from build123d import *

# Parameters (mm, degrees)
SKETCH_1_W          = 10
SKETCH_1_H          = 3
EXTRUDE_1_DEPTH     = 10
SKETCH_2_R          = 4.3
CUT_EXTRUDE_1_DEPTH = 11
SKETCH_3_R          = 1.75
CUT_EXTRUDE_2_DEPTH = 4
FILLET_1_R          = 3
FILLET_2_R          = 1


with BuildPart() as part:
    # ｽｹｯﾁ1 → ﾎﾞｽ - 押し出し1 (new body)
    with BuildSketch(Plane.XY):
        Polygon((7, 10), (1, 10), (1, -5), (7, -5), (7, 7), align=None)
        with Locations((12, 8.5)):
            Rectangle(SKETCH_1_W, SKETCH_1_H)
        Polygon((1, -5), (1, 10), (-5, 10), (-5, 7), (-5, -5), align=None)
        with Locations((-10, 8.5)):
            Rectangle(SKETCH_1_W, SKETCH_1_H)
    extrude(amount=EXTRUDE_1_DEPTH)

    # ｽｹｯﾁ2 → ｶｯﾄ - 押し出し1 (cut, through all)
    with BuildSketch(Plane(origin=(0, 0, 0), x_dir=(-1, 0, 0), z_dir=(0, 0, -1))):
        with Locations((-1, 1)):
            Circle(SKETCH_2_R)
    extrude(amount=-CUT_EXTRUDE_1_DEPTH, mode=Mode.SUBTRACT)

    # ｽｹｯﾁ3 → ｶｯﾄ - 押し出し2 (cut, through all)
    with BuildSketch(Plane.XZ.offset(-7)):
        with Locations((-11.5, 5)):
            Circle(SKETCH_3_R)
        with Locations((13.5, 5)):
            Circle(SKETCH_3_R)
    extrude(amount=-CUT_EXTRUDE_2_DEPTH, mode=Mode.SUBTRACT)

    # ﾌｨﾚｯﾄ1
    fillet_1_edges = [part.edges().sort_by_distance(p)[0] for p in [
        (7, -5, 5),
        (-5, -5, 5),
        (-5, 7, 5),
        (7, 7, 5),
    ]]
    fillet(fillet_1_edges, radius=FILLET_1_R)

    # ﾌｨﾚｯﾄ2
    fillet_2_edges = [part.edges().sort_by_distance(p)[0] for p in [
        (-15, 8.5, 0),
        (17, 8.5, 0),
        (17, 8.5, 10),
        (-15, 7, 5),
        (17, 7, 5),
        (-15, 8.5, 10),
        (-5, 1, 0),
        (-5, 1, 10),
        (-11.5, 7, 0),
        (-11.5, 7, 10),
        (13.5, 7, 0),
        (13.5, 7, 10),
        (7, 1, 0),
        (7, 1, 10),
        (1, -5, 0),
        (1, -5, 10),
        (6.121320344, -4.121320344, 0),
        (-4.121320344, -4.121320344, 0),
        (6.121320344, -4.121320344, 10),
        (-4.121320344, -4.121320344, 10),
        (-5.878679656, 6.121320344, 0),
        (-5.878679656, 6.121320344, 10),
        (7.878679656, 6.121320344, 0),
        (7.878679656, 6.121320344, 10),
    ]]
    fillet(fillet_2_edges, radius=FILLET_2_R)


solid = part.part
Work out the finished part from the listing and answer in its coordinate system (mm). A direction names the side the tool comes from. Give positions to 0.01 mm unless a question says otherwise; leave off trailing zeros. Write each loop counter-clockwise with the first axis right and the second up, starting at its lowest first coordinate (ties: lowest second). Pieces come first, ordered by that corner, then holes.
Q1. The part is cut by section A-A on z = 5. Give the vertices of the cut face in (x, y), and give its area (3 significant figures).
Answer:
outline: (-15, 8) arc R1 ccw to (-14, 7) - (-13.25, 7) - (-13.25, 10) - (-15, 10) - close; (-9.75, 7) - (-8, 7) arc R3 cw to (-5, 4) - (-5, -2) arc R3 ccw to (-2, -5) - (4, -5) arc R3 ccw to (7, -2) - (7, 4) arc R3 cw to (10, 7) - (11.75, 7) - (11.75, 10) - (-9.75, 10) - close; (15.25, 7) - (16, 7) arc R1 ccw to (17, 8) - (17, 10) - (15.25, 10) - close; hole circle Ø8.6 at (1, 1)
area: 160 mm2
Q2. The part is cut by section C-C on y = 1. Give the vertices of the cut face in (x, z), and give its area (3 significant figures).
Answer:
outline: (-5, 1) arc R1 ccw to (-4, 0) - (-3.3, 0) - (-3.3, 10) - (-4, 10) arc R1 ccw to (-5, 9) - close; (5.3, 0) - (6, 0) arc R1 ccw to (7, 1) - (7, 9) arc R1 ccw to (6, 10) - (5.3, 10) - close
area: 33.1 mm2
Q3. For a pull along X with two mould halves and no side action, classify faces 1 (the face through (17, 9, 5)), 2 (the face through (13.042, 7.301, 0.285)), 3 (the face through (14.31, 8.48, 3.45)), 4 (the face through (-5, 1, 5)) as released by +X, released by -X, zero draft, split by the parting line, or undercut.
Answer:
face 1: released by +X
face 2: zero draft
face 3: undercut
face 4: released by -X
Q4. The part is cut by section D-D on z = 2.5. Give the vertices of the cut face in (x, y), and give its area (3 significant figures).
Answer:
outline: (-15, 8) arc R1 ccw to (-14, 7) - (-8, 7) arc R3 cw to (-5, 4) - (-5, -2) arc R3 ccw to (-2, -5) - (4, -5) arc R3 ccw to (7, -2) - (7, 4) arc R3 cw to (10, 7) - (16, 7) arc R1 ccw to (17, 8) - (17, 10) - (-15, 10) - close; hole circle Ø8.6 at (1, 1)
area: 181 mm2
Q5. A tool of negligible diameter and unlimited length cuts with its end or side. For faces 5 (the face through (1, 6, 10)), 6 (the face through (-10.958, 7.301, 0.285)), 7 (the face through (11.6, 7, 4.9)), 8 (the face through (-9.7, 7, 4.1)), 9 (the face through (13.042, 7.301, 9.715)), from which of +Z, -Z, +X, -X, +Y, -Y can it reach the whole face along a straight path? Write none if from no direction.
Answer:
face 5: +Z, +X, -X, +Y, -Y
face 6: -Z, -X, -Y
face 7: +Z, -Z, +X, -Y
face 8: +Z, -Z, -X, -Y
face 9: +Z, +X, -Y
Q6. Given pin 1 (5 mm diameter, centred on y = 0, z = 5, fed in from +X); pin 2 (5 mm diameter, centred on x = 14, z = 5, fed in from -Y); pin 3 (1.5 mm diameter, centred on y = -1.5, z = 1.5, fed in from -X), each flat-ended and moving along its own axis, determine where each tip first touches the part or whether it passes through.
Answer:
pin 1: stops at x = 7
pin 2: stops at y = 7
pin 3: stops at x = -5
Q7. The part is cut by section B-B on x = 13.5. Give the vertices of the cut face in (y, z), and give its area (3 significant figures).
Answer:
outline: (7, 1) arc R1 ccw to (8, 0) - (10, 0) - (10, 3.25) - (7, 3.25) - close; (7, 6.75) - (10, 6.75) - (10, 10) - (8, 10) arc R1 ccw to (7, 9) - close
area: 19.1 mm2
Q8. Straight lines are drawn through the part: L1, parallel to Z at x = 13.5, y = 8.7; L2, parallel to Y at x = 1, z = 1.5; L3, parallel to Y at x = 10.5, z = 6. For each, find the intervals that lie inside material, in ascending order.
Answer:
L1: z = 0 to 3.25, 6.75 to 10
L2: y = -5 to -3.3, 5.3 to 10
L3: y = 7 to 10
